from build123d import *

# Parameters (mm, degrees)
SKETCH1_R               = 1.651
BOSS_EXTRUDE2_DEPTH     = 3.175
SKETCH2_R               = 1.143
CUT_EXTRUDE1_DEPTH      = 101.402396032
SKETCH3_R               = 12.1285
CUT_EXTRUDE2_DEPTH      = 101.402396032
SKETCH4_R               = 38.1
CUT_EXTRUDE3_DEPTH      = 124.46
SKETCH5_R               = 5
CUT_EXTRUDE4_DEPTH      = 101.402396032
SKETCH6_R               = 1.651
CUT_EXTRUDE5_DEPTH      = 223.668813424
SKETCH7_R               = 3.175
CUT_EXTRUDE6_DEPTH      = 226.368754426
CUT_EXTRUDE6_DEPTH_BACK = 226.368754426
FILLET1_R               = 6.35
SKETCH8_R               = 1.651
CUT_EXTRUDE7_DEPTH      = 29.21
SKETCH9_R               = 3.5
CUT_EXTRUDE8_DEPTH      = 101.402396176


with BuildPart() as part:
    # Sketch1 → Boss-Extrude2 (new body)
    with BuildSketch(Plane.XY):
        with BuildLine():
            Line((-66.753693561, 34.036), (-54.815693561, 34.036))
            Line((-54.815693561, 34.036), (-54.815693561, -34.036))
            Line((-54.815693561, -34.036), (-66.753693561, -34.036))
            ThreePointArc((-66.753693561, -34.036), (0, -74.93), (66.753693561, -34.036))
            Line((66.753693561, -34.036), (54.815693561, -34.036))
            Line((54.815693561, -34.036), (54.815693561, 34.036))
            Line((54.815693561, 34.036), (66.753693561, 34.036))
            ThreePointArc((66.753693561, 34.036), (0, 74.93), (-66.753693561, 34.036))
        make_face()
        with Locations((-46.482, 10.795)):
            Circle(SKETCH1_R, mode=Mode.SUBTRACT)
        with Locations((-21.082, 10.795)):
            Circle(SKETCH1_R, mode=Mode.SUBTRACT)
        with Locations(Location((-21.082, -10.795, 0), (0, 0, 180))):
            Circle(SKETCH1_R, mode=Mode.SUBTRACT)
        with Locations(Location((-46.482, -10.795, 0), (0, 0, 180))):
            Circle(SKETCH1_R, mode=Mode.SUBTRACT)
        with Locations((46.482, -10.795)):
            Circle(SKETCH1_R, mode=Mode.SUBTRACT)
        with Locations((21.082, -10.795)):
            Circle(SKETCH1_R, mode=Mode.SUBTRACT)
        with Locations(Location((21.082, 10.795, 0), (0, 0, 180))):
            Circle(SKETCH1_R, mode=Mode.SUBTRACT)
        with Locations(Location((46.482, 10.795, 0), (0, 0, 180))):
            Circle(SKETCH1_R, mode=Mode.SUBTRACT)
    extrude(amount=BOSS_EXTRUDE2_DEPTH)

    # Sketch2 → Cut-Extrude1 (cut, through all)
    with BuildSketch(Plane.XY.offset(3.175)):
        with Locations((-6.731, 62.23)):
            Circle(SKETCH2_R)
        with Locations(Location((6.731, 62.23, 0), (0, 0, 180))):
            Circle(SKETCH2_R)
    extrude(amount=-CUT_EXTRUDE1_DEPTH, mode=Mode.SUBTRACT)

    # Sketch3 → Cut-Extrude2 (cut, through all)
    with BuildSketch(Plane(origin=(0, 0, 0), x_dir=(-1, 0, 0), z_dir=(0, 0, -1))):
        with Locations((0, -13.208)):
            Circle(SKETCH3_R)
        with Locations((0, 13.208)):
            Circle(SKETCH3_R)
        with Locations((-43.105229381, -43.105229381)):
            Circle(SKETCH3_R)
        with Locations((19.05, -32.995567884)):
            Circle(SKETCH3_R)
        with Locations(Location((19.05, 32.995567884, 0), (0, 0, 180))):
            Circle(SKETCH3_R)
        with Locations((-43.105229381, 43.105229381)):
            Circle(SKETCH3_R)
        with Locations((43.105229381, 43.105229381)):
            Circle(SKETCH3_R)
        with Locations((-19.05, 32.995567884)):
            Circle(SKETCH3_R)
        with Locations(Location((-19.05, -32.995567884, 0), (0, 0, 180))):
            Circle(SKETCH3_R)
        with Locations((43.105229381, -43.105229381)):
            Circle(SKETCH3_R)
    extrude(amount=-CUT_EXTRUDE2_DEPTH, mode=Mode.SUBTRACT)

    # Sketch4 → Cut-Extrude3 (cut)
    with BuildSketch(Plane(origin=(0, 0, 0), x_dir=(-1, 0, 0), z_dir=(0, 0, -1))):
        with Locations((0, -86.312058398)):
            Circle(SKETCH4_R)
    extrude(amount=-CUT_EXTRUDE3_DEPTH, mode=Mode.SUBTRACT)

    # Sketch5 → Cut-Extrude4 (cut, through all)
    with BuildSketch(Plane(origin=(0, 0, 0), x_dir=(-1, 0, 0), z_dir=(0, 0, -1))):
        with Locations((34.798, -15.24)):
            Circle(SKETCH5_R)
        with Locations(Location((-34.798, -15.24, 0), (0, 0, 180))):
            Circle(SKETCH5_R)
        with Locations((-34.798, 15.24)):
            Circle(SKETCH5_R)
        with Locations(Location((34.798, 15.24, 0), (0, 0, 180))):
            Circle(SKETCH5_R)
    extrude(amount=-CUT_EXTRUDE4_DEPTH, mode=Mode.SUBTRACT)

    # Sketch6 → Cut-Extrude5 (cut, through all)
    with BuildSketch(Plane(origin=(31.313436391, 132.613959999, 0), x_dir=(0, 1, 0), z_dir=(0, 0, -1))):
        with Locations(Location((-180.873959999, -4.643436391, 0), (0, 0, 270))):
            Circle(SKETCH6_R)
        with Locations(Location((-180.873959999, -57.983436391, 0), (0, 0, 90))):
            Circle(SKETCH6_R)
        with Locations(Location((-84.353959999, -57.983436391, 0), (0, 0, 270))):
            Circle(SKETCH6_R)
        with Locations(Location((-84.353959999, -4.643436391, 0), (0, 0, 90))):
            Circle(SKETCH6_R)
    extrude(amount=-CUT_EXTRUDE5_DEPTH, mode=Mode.SUBTRACT)

    # Sketch7 → Cut-Extrude6 (cut, two sides)
    with BuildSketch(Plane(origin=(31.313436391, 132.613959999, -31.75), x_dir=(0, 1, 0), z_dir=(0, 0, -1))) as cut_extrude6_sk:
        with Locations((-158.013959999, 14.406563609)):
            Circle(SKETCH7_R)
        with Locations((-169.443959999, -31.313436391)):
            Circle(SKETCH7_R)
        with Locations((-158.013959999, -77.033436391)):
            Circle(SKETCH7_R)
        with Locations((-107.213959999, -77.033436391)):
            Circle(SKETCH7_R)
        with Locations((-95.783959999, -31.313436391)):
            Circle(SKETCH7_R)
        with Locations((-107.213959999, 14.406563609)):
            Circle(SKETCH7_R)
    extrude(amount=CUT_EXTRUDE6_DEPTH, mode=Mode.SUBTRACT)
    extrude(cut_extrude6_sk.sketch, amount=-CUT_EXTRUDE6_DEPTH_BACK, mode=Mode.SUBTRACT)

    # Fillet1
    fillet1_edges = [part.edges().sort_by_distance(p)[0] for p in [
        (33.000960548, -67.271401821, 1.5875),
        (-33.000960548, -67.271401821, 1.5875),
    ]]
    fillet(fillet1_edges, radius=FILLET1_R)

    # Sketch8 → Cut-Extrude7 (cut)
    with BuildSketch(Plane(origin=(31.313436391, 132.613959999, -28.575), x_dir=(0, 1, 0), z_dir=(0, 0, -1))):
        with Locations(Location((-191.033959999, 2.976563609, 0), (0, 0, 270))):
            Circle(SKETCH8_R)
        with Locations(Location((-191.033959999, -65.603436391, 0), (0, 0, 270))):
            Circle(SKETCH8_R)
        with Locations(Location((-74.193959999, -65.603436391, 0), (0, 0, 270))):
            Circle(SKETCH8_R)
        with Locations(Location((-74.193959999, 2.976563609, 0), (0, 0, 270))):
            Circle(SKETCH8_R)
    extrude(amount=-CUT_EXTRUDE7_DEPTH, mode=Mode.SUBTRACT)

    # Sketch9 → Cut-Extrude8 (cut, through all)
    with BuildSketch(Plane(origin=(0, 0, 0), x_dir=(-1, 0, 0), z_dir=(0, 0, -1))):
        with Locations((34.29, 58.42)):
            Circle(SKETCH9_R)
        with Locations((-34.29, 58.42)):
            Circle(SKETCH9_R)
        with Locations((-34.29, -58.42)):
            Circle(SKETCH9_R)
        with Locations((34.29, -58.42)):
            Circle(SKETCH9_R)
    extrude(amount=-CUT_EXTRUDE8_DEPTH, mode=Mode.SUBTRACT)


solid = part.part
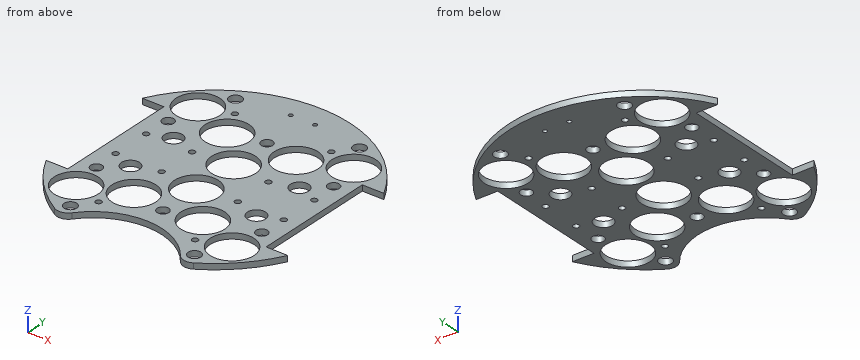
CAD build for the part. Positions are in the model's coordinates, mm. Coordinates: 2 decimals unless noted, no trailing zeros. Loops run counter-clockwise (first coordinate to the right, second up) from the corner with the lowest first, then second, coordinate; pieces in that order, holes last. Notation, with made-up numbers: (62, -39.5) - (78, -39.5) arc R16 ccw to (78, -23.5) - close; hole circle Ø10 at (4.5, 15). An arc over 180 degrees is marked (long way). Use one line per item in the form item = value. Start each with the question number.
1) Drill centre lines: L1, parallel to Y at x = -19.05, z = 1.55; L2, parallel to X at y = -36, z = 2.85; L3, parallel to Y at x = 51, z = 0.8. Where is each one in solid material? Low to high. Write a range as from..to.
2) Band-saw the part on B-B (y = 36.83). Give the cut face in (x, z) (3 decimals).
3) Band-saw the part on A-A (x = -26.67). Give the cut face in (y, z) (3 decimals).
4) Flat gauge pins, fed straight in: pin 1 (3 mm diameter, centred on x = 21.082, y = 10.795, fed in from +Z); pin 2 (1.6 mm diameter, centred on y = 0, z = 1.5, fed in from -X). Where does each tip first touch, or does it go through?
5) Band-saw the part on C-C (y = 58.42). Give the cut face in (x, z) (3 decimals), and give its area (4 significant figures).
6) Band-saw the part on D-D (x = -53). Give the cut face in (y, z) (3 decimals).
Check values:
q1.L1 = -53.32..-45.12, -20.87..20.87, 45.12..72.47
q1.L2 = -65.72..-52.93, -33.28..-30.8, -7.3..-3.06, 3.06..7.3, 30.8..33.28, 52.93..65.72
q1.L3 = -54.9..-52.31, -33.9..33.9, 52.31..54.9
q2.outline = (-65.254, 0) - (-53.484, 0) - (-53.484, 3.175) - (-65.254, 3.175) - close; (-32.726, 0) - (-30.556, 0) - (-30.556, 3.175) - (-32.726, 3.175) - close; (-7.544, 0) - (-3.175, 0) - (-3.175, 3.175) - (-7.544, 3.175) - close; (3.175, 0) - (7.544, 0) - (7.544, 3.175) - (3.175, 3.175) - close; (30.556, 0) - (32.726, 0) - (32.726, 3.175) - (30.556, 3.175) - close; (53.484, 0) - (65.254, 0) - (65.254, 3.175) - (53.484, 3.175) - close
q3.outline = (-59.103, 0) - (-49.911, 0) - (-49.911, 3.175) - (-59.103, 3.175) - close; (-46.609, 0) - (-42.431, 0) - (-42.431, 3.175) - (-46.609, 3.175) - close; (-23.56, 0) - (23.56, 0) - (23.56, 3.175) - (-23.56, 3.175) - close; (42.431, 0) - (46.609, 0) - (46.609, 3.175) - (42.431, 3.175) - close; (49.911, 0) - (70.023, 0) - (70.023, 3.175) - (49.911, 3.175) - close
q4.pin_1 = through
q4.pin_2 = -54.82
q5.outline = (-46.921, 0) - (-37.79, 0) - (-37.79, 3.175) - (-46.921, 3.175) - close; (-30.79, 0) - (30.79, 0) - (30.79, 3.175) - (-30.79, 3.175) - close; (37.79, 0) - (46.921, 0) - (46.921, 3.175) - (37.79, 3.175) - close
q5.area = 253.5 mm2
q6.outline = (-52.967, 0) - (-50.119, 0) - (-50.119, 3.175) - (-52.967, 3.175) - close; (-36.091, 0) - (36.091, 0) - (36.091, 3.175) - (-36.091, 3.175) - close; (50.119, 0) - (52.967, 0) - (52.967, 3.175) - (50.119, 3.175) - close
